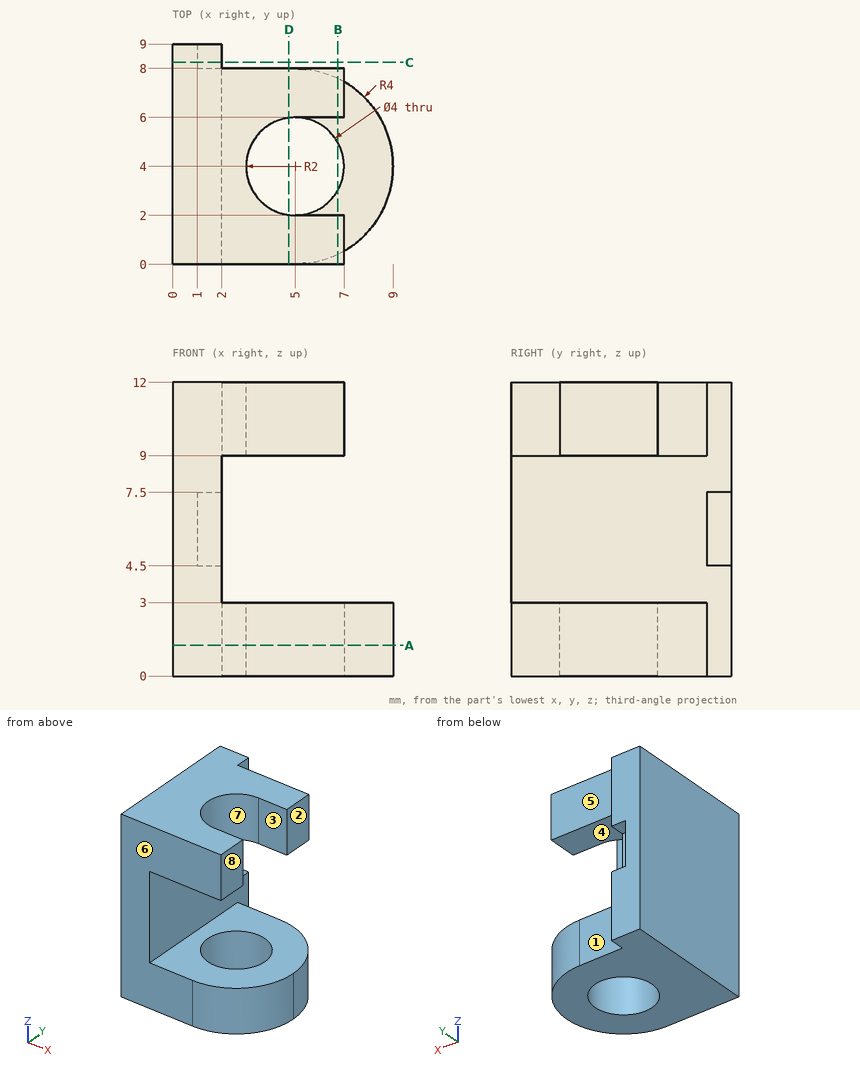
Answer from the drawing. Dimensions are ordinates in mm from the lowest x, y and z of the part. A direction names the side the tool comes from. Round coordinates to 2 decimals unless told otherwise and drop trailing zeros. Order: outer loops, then holes, each group sorted by start corner. A loop starts at its lowest first (then second) coordinate and runs counter-clockwise, first axis right, second up.
1) The mould has two halves that part along Y. Classify the marked faces 5, 6, 7 and 8: released by +Y, released by -Y, zero draft, split by the parting line, or undercut.
2) Flat-ended cylindrical pins translate along their axes: pin 1 (4 mm diameter, centred on x = 3.5, y = 3.5, fed in from +Z); pin 2 (2 mm diameter, centred on y = 6.5, z = 6.5, fed in from +X); pin 3 (1 mm diameter, centred on x = 6.5, z = 10.5, fed in from +Y); pin 4 (0.6 mm diameter, centred on y = 0.5, z = 11, fed in from +X). Find the tip coordinate at first contact, or state that the pin passes through.
3) The part is cut by section A-A on z = 1.25. Write down the section's boundary in (x, y).
4) For the marked faces 1, 2, 3 and 4, determine the directions among +Z, -Z, +X, -X, +Y, -Y from which every point of the face is accessible in a straight line to the end or side of a thin tool.
5) The part is cut by section C-C on y = 8.25. Write down the section's boundary in (x, z), plus the area to 3 significant figures.
6) The part is cut by section B-B on x = 6.75. Write down the section's boundary in (y, z).
7) Straight lines are drawn through the part: L1, parallel to Y at x = 5.5, z = 9.75; L2, parallel to Z at x = 5.5, y = 7.25; L3, parallel to Z at x = 7.75, y = 1.25. For each, find the intervals that lie inside material, in ascending order.
8) The part is cut by section D-D on x = 4.75. Write down the section's boundary in (y, z), plus the area to 3 significant figures.
Resolved:
1. face 5: released by +Y
1. face 6: released by -Y
1. face 7: undercut
1. face 8: zero draft
2. pin 1: stops at z = 12
2. pin 2: stops at x = 2
2. pin 3: stops at y = 8
2. pin 4: stops at x = 7
3. outline: (0, 0) - (5, 0) arc R4 ccw to (5, 8) - (2, 8) - (2, 9) - (0, 9) - close; hole circle Ø4 at (5, 4)
4. face 1: +Z, -Z, +X, +Y
4. face 2: +Z, +X, +Y, -Y
4. face 3: +Z, +X
4. face 4: +X, +Y, -Y
5. outline: (0, 0) - (2, 0) - (2, 4.5) - (1, 4.5) - (1, 7.5) - (2, 7.5) - (2, 12) - (0, 12) - close
5. area: 21.0 mm2
6. outline: (0, 9) - (2, 9) - (2, 12) - (0, 12) - close; (0.4, 0) - (3.03, 0) - (3.03, 3) - (0.4, 3) - close; (4.97, 0) - (7.6, 0) - (7.6, 3) - (4.97, 3) - close; (6, 9) - (8, 9) - (8, 12) - (6, 12) - close
7. L1: y = 0 to 2, 6 to 8
7. L2: z = 0 to 3, 9 to 12
7. L3: z = 0 to 3
8. outline: (0, 0) - (2.02, 0) - (2.02, 3) - (0, 3) - close; (0, 9) - (2.02, 9) - (2.02, 12) - (0, 12) - close; (5.98, 0) - (8, 0) - (8, 3) - (5.98, 3) - close; (5.98, 9) - (8, 9) - (8, 12) - (5.98, 12) - close
8. area: 24.2 mm2
